For this review, take the finished solid that the model builds, in its own axes (mm). Give positions to 0.01 mm unless a question says otherwise; leave off trailing zeros. Write each loop counter-clockwise with the first axis right and the second up, starting at its lowest first coordinate (ties: lowest second). Pieces come first, ordered by that corner, then holes. Notation, with made-up numbers: (13.5, 61) -> (33.5, 61) arc R22 ccw to (33.5, 86) -> close; hole circle Ø3 at (-37.75, -6). An arc over 180 degrees is marked (long way). Write item = value, one per line.
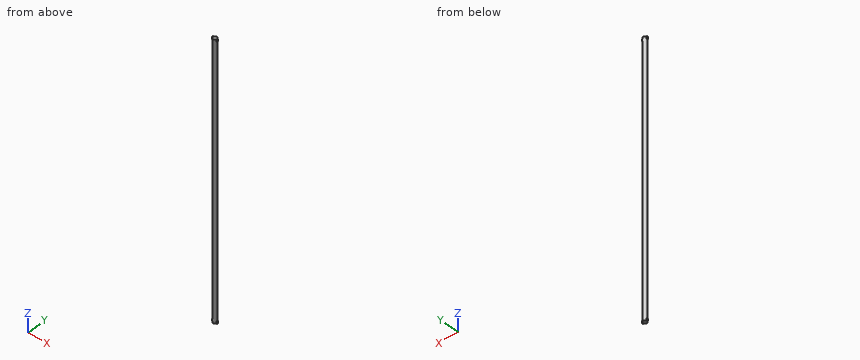
```python
from build123d import *

# Parameters (mm, degrees)
SKETCH1_R              = 3.175
BOSS_EXTRUDE1_DEPTH    = 457.2
BOSS_EXTRUDE2_START    = -3.81
BOSS_EXTRUDE2_DEPTH    = 3.81
CIRPATTERN1_COUNT      = 2
LPATTERN1_COUNT        = 2
LPATTERN1_PITCH        = 453.39
LPATTERN1_START        = -3.81
LPATTERN1_COPY_1_DEPTH = 3.81


with BuildPart() as part:
    # Sketch1 → Boss-Extrude1 (new body)
    with BuildSketch(Plane.XY):
        Circle(SKETCH1_R)
    extrude(amount=BOSS_EXTRUDE1_DEPTH)

    # Sketch3 → Boss-Extrude2 (add)
    with BuildSketch(Plane.XY.offset(457.2).offset(BOSS_EXTRUDE2_START)):
        with BuildLine():
            Line((4.445, 0.9525), (4.445, -0.9525))
            Line((4.445, -0.9525), (3.028756964, -0.9525))
            ThreePointArc((3.028756964, -0.9525), (3.175, 0), (3.028756964, 0.9525))
            Line((3.028756964, 0.9525), (4.445, 0.9525))
        make_face()
    boss_extrude2 = extrude(amount=BOSS_EXTRUDE2_DEPTH)

    # CirPattern1: Boss-Extrude2 ×2 about axis
    cirpattern1_axis = Axis((0, 0, 0), (0, 0, 1))
    for i in range(1, CIRPATTERN1_COUNT):
        add(boss_extrude2.rotate(cirpattern1_axis, i * 360 / CIRPATTERN1_COUNT))

    # LPattern1: Boss-Extrude2 ×2
    with Locations(*[(0, 0, -i * LPATTERN1_PITCH) for i in range(1, LPATTERN1_COUNT)]):
        add(boss_extrude2)

    # LPattern1 copy 1 sketch → LPattern1 copy 1 (add)
    with BuildSketch(Plane(origin=(0, 0, 3.81), x_dir=(-1, 0, 0), z_dir=(0, 0, 1)).offset(LPATTERN1_START)):
        with BuildLine():
            Line((4.445, 0.9525), (4.445, -0.9525))
            Line((4.445, -0.9525), (3.028756964, -0.9525))
            ThreePointArc((3.028756964, -0.9525), (3.175, 0), (3.028756964, 0.9525))
            Line((3.028756964, 0.9525), (4.445, 0.9525))
        make_face()
    extrude(amount=LPATTERN1_COPY_1_DEPTH)


solid = part.part
```
(1) To check wall thickness, follow probe 1 along Z at (x, y) = (3.5, 0.5); probe 2 along X at (y, z) = (1, 388); probe 3 along X at (y, z) = (0.25, 344.5). State the ranges of each line that lie inside material, in increasing order.
Answers below:
probe_1 = 0 to 3.81, 453.39 to 457.2
probe_2 = -3.01 to 3.01
probe_3 = -3.17 to 3.17
(2) Take a section at A-A (z = 105). Write out the cut boundary in (x, y) (3 decimals).
Answers below:
outline = circle Ø6.35 at (0, 0)
(3) Take a section at B-B (x = -1). Write out the cut boundary in (y, z), plus the area to 3 significant figures.
Answers below:
outline = (-3.01, 0) -> (3.01, 0) -> (3.01, 457.2) -> (-3.01, 457.2) -> close
area = 2,760 mm^2
(4) For pin 1 (1.6 mm diameter, centred on x = 3.5, z = 1, fed in from -Y); pin 2 (3 mm diameter, centred on y = 1, z = 230, fed in from +X) (3 decimals); pin 3 (1.6 mm diameter, centred on x = 3.5, z = 1.5, fed in from +Y), all flat-tipped, find the tip position at first contact; note any pin that passes through.
Answers below:
pin_1 = -1.67
pin_2 = 3.175
pin_3 = 1.67
